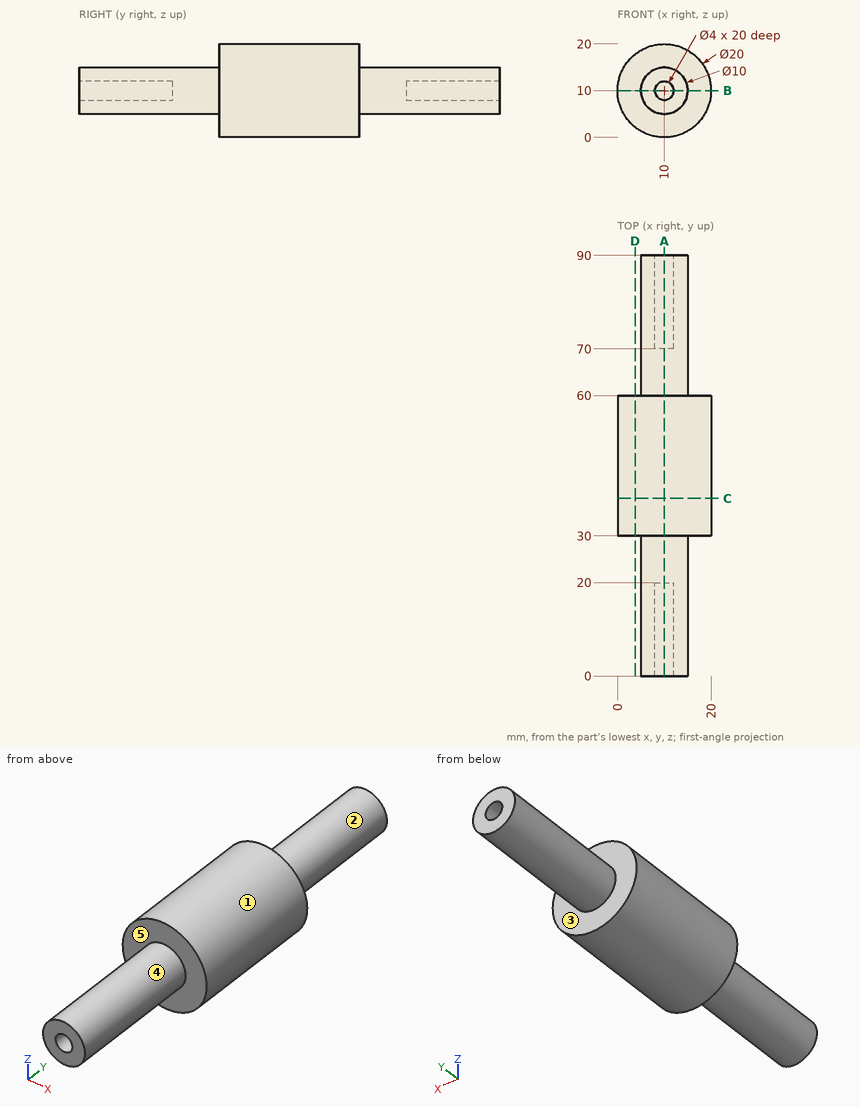
Design review of the part shown in the three views and the two pictorial views. Dimensions are in mm from the part's minimum x, y and z. A direction names the side the tool comes from. Coordinates: 2 decimals unless noted, no trailing zeros. Loops run counter-clockwise (first coordinate to the right, second up) from the corner with the lowest first, then second, coordinate; pieces in that order, holes last. Notation, with made-up numbers: (-16, 11.5) - (26, 11.5) arc R22 ccw to (26, 23.5) - close; hole circle Ø6 at (16, 64.25). An arc over 180 degrees is marked (long way). Use a Markdown table: item, result. Add a question column.
Item 1: Insertion check: pin 1 Ø1 at (x, y) = (4, 45.5) entering from -Z; pin 2 Ø2 at (x, y) = (2.5, 34) entering from +Z; pin 3 Ø2 at (x, z) = (10, 9.5) entering from +Y. Each pin has a flat end and moves straight along its axis. Give the tip position at first contact, or say it passes through.
Item 2: We need section B-B (z = 10). Give the boundary of the cut face in (x, y).
Item 3: For line 1 (X direction, y = 82.75, z = 10); line 2 (Y direction, x = 3.5, z = 16.25); line 3 (Y direction, x = 11.5, z = 11.25), list the stretches that pass through material, from the lowest coordinate up.
Item 4: Tool access review of the marked faces 1 and 2: name each direction out of +Z, -Z, +X, -X, +Y, -Y from which nothing blocks a thin tool from reaching the whole face with its end or side.
Item 5: We need section A-A (x = 10). Give the boundary of the cut face in (y, z), and give its area (3 significant figures).
Item 6: We need section D-D (x = 3.75). Give the boundary of the cut face in (y, z), and give its area (3 significant figures).
Item 7: Mouldability with a two-part tool opening along Y and no side actions: class the marked faces 3, 4 and 5 as pulls with the +Y half, pulls with the -Y half, needs draft (parallel to the pull), parting line crosses it, or undercut.
Item 8: We need section C-C (y = 38). Give the boundary of the cut face in (x, z).
Results list:
| question | item | result |
|---|---|---|
| 1 | pin 1 | stops at z = 1.65 |
| 1 | pin 2 | stops at z = 17.6 |
| 1 | pin 3 | stops at y = 70 |
| 2 | outline | (0, 30) - (5, 30) - (5, 0) - (8, 0) - (8, 20) - (12, 20) - (12, 0) - (15, 0) - (15, 30) - (20, 30) - (20, 60) - (15, 60) - (15, 90) - (12, 90) - (12, 70) - (8, 70) - (8, 90) - (5, 90) - (5, 60) - (0, 60) - close |
| 3 | line 1 | x = 5 to 8, 12 to 15 |
| 3 | line 2 | y = 30 to 60 |
| 3 | line 3 | y = 20 to 70 |
| 4 | face 1 | +Y, -Y |
| 4 | face 2 | +Y |
| 5 | outline | (0, 5) - (30, 5) - (30, 0) - (60, 0) - (60, 5) - (90, 5) - (90, 8) - (70, 8) - (70, 12) - (90, 12) - (90, 15) - (60, 15) - (60, 20) - (30, 20) - (30, 15) - (0, 15) - (0, 12) - (20, 12) - (20, 8) - (0, 8) - close |
| 5 | area | 1,040 mm^2 |
| 6 | outline | (30, 2.19) - (60, 2.19) - (60, 17.81) - (30, 17.81) - close |
| 6 | area | 468 mm^2 |
| 7 | face 3 | pulls with the +Y half |
| 7 | face 4 | needs draft |
| 7 | face 5 | pulls with the -Y half |
| 8 | outline | circle Ø20 at (10, 10) |
